Job drawing, mm, ordinate dimensions from the low corner. One solid piece. A direction names the side the tool comes from. Give positions to 0.01 mm unless a question says otherwise; leave off trailing zeros. Loops run counter-clockwise (first coordinate to the right, second up) from the corner with the lowest first, then second, coordinate; pieces in that order, holes last. Notation, with made-up numbers: M -16.5,65.5 L 30.5,65.5 A12 cw 30.5,87.5 Z; hole C -19,66.5 d2. An arc over 180 degrees is marked long. Put each result on its own line as item: value.
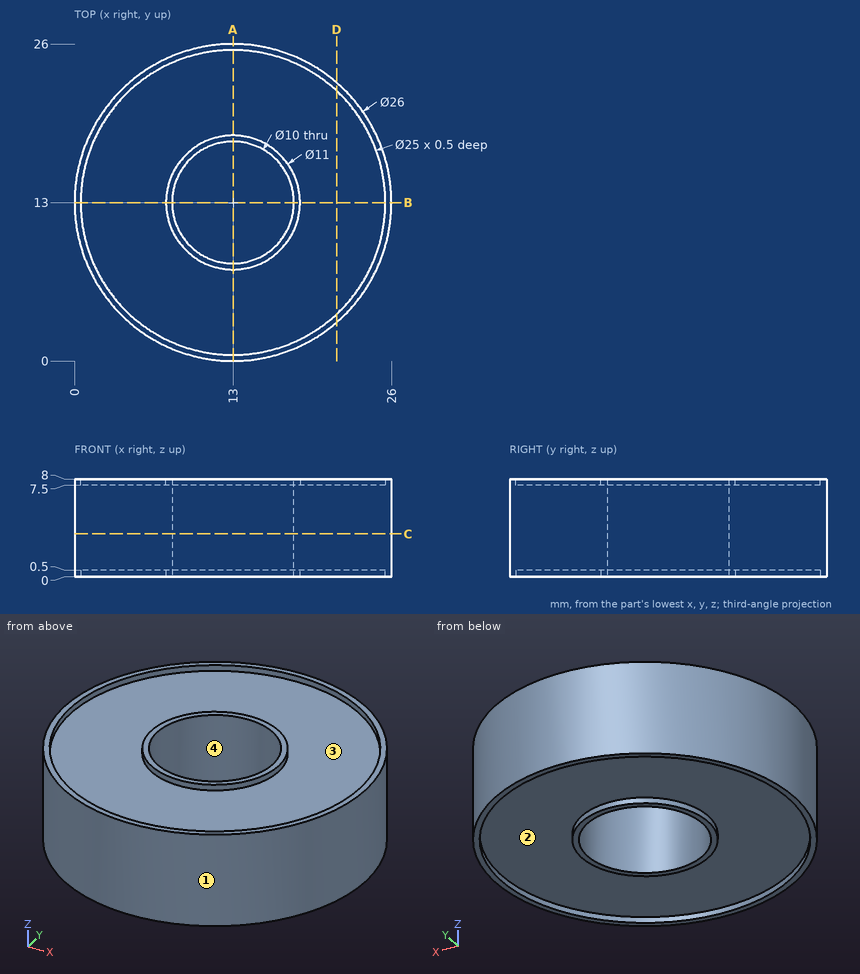
Q1. Mould opens along Y. For the marked faces 1 and 2 say: pulls with the +Y half, pulls with the -Y half, needs draft (parallel to the pull), parting line crosses it, or undercut.
Here are the results:
face 1: parting line crosses it
face 2: undercut
Q2. Slice it at A-A (x = 13). List the corners of the cut face in (y, z), and give its area (3 significant figures).
Here are the results:
outline: M 0,0 L 0.5,0 L 0.5,0.5 L 7.5,0.5 L 7.5,0 L 8,0 L 8,8 L 7.5,8 L 7.5,7.5 L 0.5,7.5 L 0.5,8 L 0,8 Z; M 18,0 L 18.5,0 L 18.5,0.5 L 25.5,0.5 L 25.5,0 L 26,0 L 26,8 L 25.5,8 L 25.5,7.5 L 18.5,7.5 L 18.5,8 L 18,8 Z
area: 114 mm²
Q3. Drop flat-ended pins along their axis: pin 1 Ø3 at (x, z) = (3, 6) entering from -Y; pin 2 Ø1 at (y, z) = (5.5, 3.5) entering from -X; pin 3 Ø1 at (y, z) = (4, 6) entering from +X; pin 4 Ø9 at (x, y) = (13, 13) entering from -Z. Give the stop position or say it passes through.
Here are the results:
pin 1: y = 3.16
pin 2: x = 2.05
pin 3: x = 22.84
pin 4: through
Q4. Probe line 1 (Y direction, x = 13, z = 0.45); line 2 (Y direction, x = 13, z = 5.5); line 3 (Z direction, x = 18.25, y = 11.25). List the from-to ranges inside material, lowest first. Write a range as from..to.
Here are the results:
line 1: 0..0.5, 7.5..8, 18..18.5, 25.5..26
line 2: 0..8, 18..26
line 3: 0.5..7.5
Q5. Tool access for the marked faces 3 and 4: list every direction of +Z, -Z, +X, -X, +Y, -Y with a clear straight run to the whole face (end or side of a thin tool).
Here are the results:
face 3: +Z
face 4: +Z, -Z
Q6. Slice it at D-D (x = 21.5). List the corners of the cut face in (y, z), and give its area (3 significant figures).
Here are the results:
outline: M 3.16,0 L 3.83,0 L 3.83,0.5 L 22.17,0.5 L 22.17,0 L 22.84,0 L 22.84,8 L 22.17,8 L 22.17,7.5 L 3.83,7.5 L 3.83,8 L 3.16,8 Z
area: 139 mm²
Q7. Slice it at C-C (z = 3.5). List the corners of the cut face in (x, y), and give its area (3 significant figures).
Here are the results:
outline: C 13,13 d26; hole C 13,13 d10
area: 452 mm²
